Autodesk Inventor part; units mm, degrees
ref_plane "YZ Plane" through (0, 0, 0) normal (1, 0, 0) x (0, 1, 0)
ref_plane "XZ Plane" through (0, 0, 0) normal (0, 1, 0) x (-1, 0, 0)
ref_plane "XY Plane" through (0, 0, 0) normal (0, 0, 1) x (1, 0, 0)
sketch "Sketch3" plane through (0, 0, 0) normal (0, 0, 1) x (1, 0, 0)
  line L0 (0, 0) -> (-10, 0)
  line L1 (-25, 0) -> (-25, 5)
  line L2 (-25, 5) -> (-15, 5)
  line L3 (-15, 5) -> (-15, 20)
  line L4 (-15, 20) -> (-10, 20)
  line L5 (0, 20) -> (0, 0)
  line L6 (0, 20) -> (-10, 20)
  line L7 (-10, 20) -> (-10, 0)
  line L8 (-10, 20) -> (0, 20)
  line L9 (-10, 0) -> (-25, 0)
  line L10 (-25, 5) -> (-25, 20)
  line L11 (-25, 20) -> (-15, 20)
  dimension "d12" = 25
  dimension "d13" = 5
  dimension "d14" = 10
  dimension "d15" = 15
  dimension "d16" = 15
  dimension "d19" = 10
extrude "Extrusion1" add sketch "Sketch3" along normal blind 15 contours L0 L7 L6 L5 | L9 L1 L2 L3 L4 L7
extrude "Extrusion2" add sketch "Sketch3" against normal blind 15 contours L9 L1 L2 L3 L4 L7 | L3 L2 L10 L11
sketch "Sketch4" plane through (-15, 20, 15) normal (0, 1, 0) x (1, 0, 0)
  line L0 (-10, 15) -> (-10, 30)
  line L1 (0, 15) -> (-10, 15)
  line L2 (-10, 15) -> (0, 0)
  line L3 (0, 0) -> (0, 15)
  point P0 (15, 15)
extrude "Extrusion3" add sketch "Sketch4" against normal blind 5
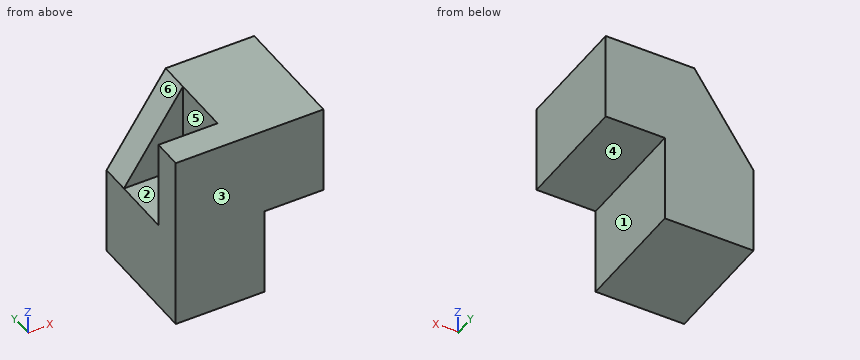
Can you work these out from the model? Positions are in its coordinate system, mm. Face numbers are marked on the shaded views. A direction names the side the tool comes from. Coordinates: 2 decimals unless noted, no trailing zeros. Order: outer loops, then holes, each group sorted by start corner. A loop starts at its lowest first (then second) coordinate and runs counter-clockwise, first axis right, second up. Notation, with made-up numbers: M 48.5,64.5 L 64.5,64.5 A13 cw 64.5,83.5 Z; hole C -37,-8.5 d1. An arc over 180 degrees is marked long. Write item = value, one per line.
(1) Suppose I cut it at C-C on y = 16.5. Please give me the cut outline in (x, z).
Results are:
outline = M -25,-15 L -10,-15 L -10,0 L 0,0 L 0,15 L -15,15 L -25,0 Z
(2) If we mould it in two halves opening along Y, with no side actions, what happens to the marked faces 1, 2 and 3? For each: pulls with the +Y half, pulls with the -Y half, needs draft (parallel to the pull), parting line crosses it, or undercut.
Results are:
face_1 = needs draft
face_2 = undercut
face_3 = pulls with the -Y half
(3) For the marked faces 4, 5 and 6, which set-ups out of +Z, -Z, +X, -X, +Y, -Y let a thin tool reach every point of the face, with its end or its side?
Results are:
face_4 = -Z, +X, +Y, -Y
face_5 = +Z, -X
face_6 = +Z, -X, +Y
(4) Suppose I cut it at D-D on x = -6. Please give me the cut outline in (y, z).
Results are:
outline = M 0,0 L 20,0 L 20,15 L 0,15 Z
(5) Suppose I cut it at B-B on z = 12.75. Please give me the cut outline in (x, y), plus the area to 4 significant figures.
Results are:
outline = M -25,0 L 0,0 L 0,20 L -16.5,20 L -16.5,15 L -15,15 L -15,5 L -25,5 Z
area = 357.5 mm2
(6) Suppose I cut it at A-A on y = 10.25. Please give me the cut outline in (x, z), plus the area to 3 significant figures.
Results are:
outline = M -25,-15 L -10,-15 L -10,0 L 0,0 L 0,15 L -15,15 L -15,0 L -25,0 Z
area = 450 mm2
(7) For pin 1 Ø2 at (x, y) = (-6, 2.5) entering from -Z; pin 2 Ø12 at (y, z) = (15, -10) entering from +X; pin 3 Ø3 at (x, z) = (-19.5, 10.5) entering from +Y; pin 4 Ø5 at (y, z) = (16.5, 5.5) entering from -X, each with a flat end and sliding along its axis, tell me the tip position at first contact or that it passes through.
Results are:
pin_1 = 0
pin_2 = -10
pin_3 = 20
pin_4 = -23
(8) I need wall thicknesses on line 1 along Y through (x, z) = (-17.5, 0.75); line 2 along Z through (x, y) = (-8.25, 19.25); line 3 along Y through (x, z) = (-23.75, 7.75). Which ranges of each line are inside material? Lowest first, please. Write a range as [from, to].
Results are:
line_1 = [0, 5], [15, 20]
line_2 = [0, 15]
line_3 = [0, 5]
